Could you check a few things on this drawing? It's one solid part, dimensions in mm from its lowest x, y, z. A direction names the side the tool comes from. Give positions to 0.01 mm unless a question says otherwise; leave off trailing zeros. Loops run counter-clockwise (first coordinate to the right, second up) from the corner with the lowest first, then second, coordinate; pieces in that order, holes last. Notation, with made-up numbers: (29.25, 42) - (36.25, 42) arc R15 ccw to (36.25, 65) - close; hole circle Ø5 at (-22, 64.25). An arc over 180 degrees is marked (long way). Write item = value, one per line.
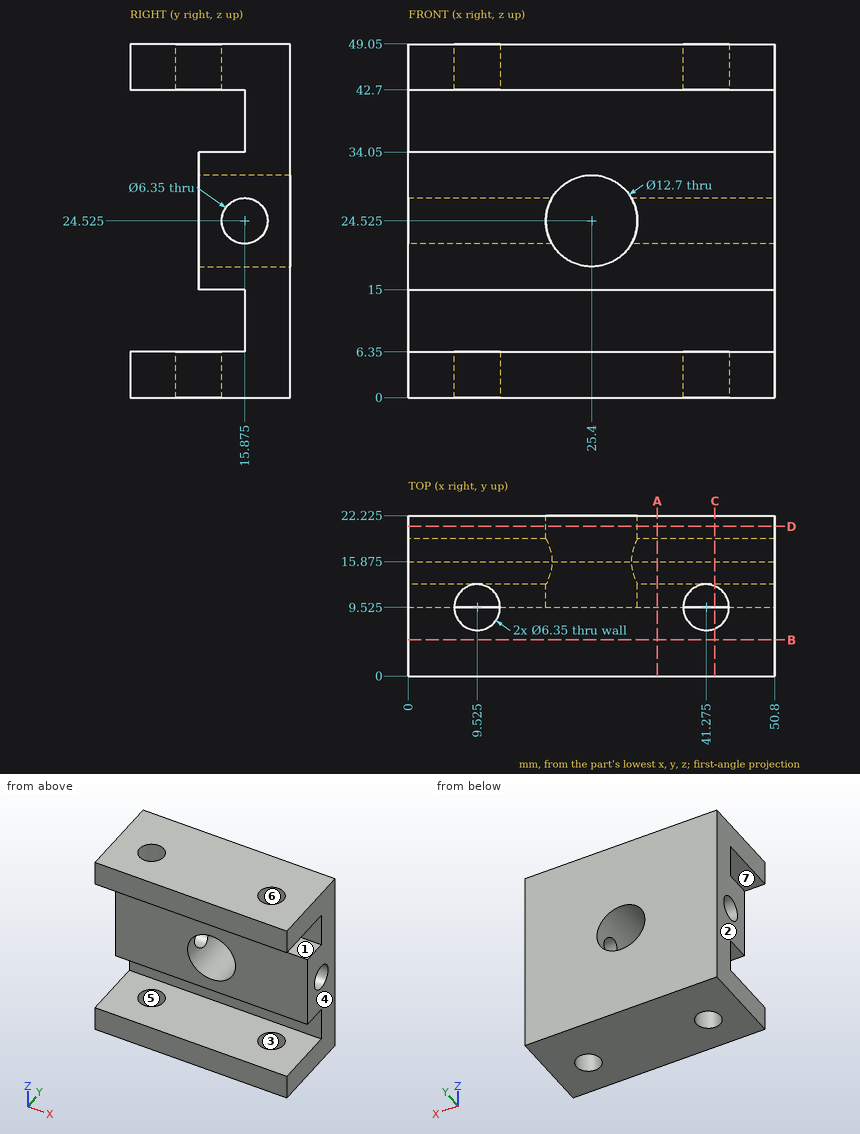
Q1. We'd pull the mould along X, two halves only. Please class the marked faces 1, 2, 3 and 4: released by +X, released by -X, zero draft, split by the parting line, or undercut.
Output:
face_1 = zero draft
face_2 = released by -X
face_3 = undercut
face_4 = released by +X
Q2. Imagine slicing it at B-B, the plane y = 5. Write out the boundary of the cut face in (x, z), then the cut area to 3 significant figures.
Output:
outline = (0, 0) - (50.8, 0) - (50.8, 6.35) - (0, 6.35) - close; (0, 42.7) - (50.8, 42.7) - (50.8, 49.05) - (0, 49.05) - close
area = 645 mm2
Q3. Which directions (+Z, -Z, +X, -X, +Y, -Y) give clear straight access to the entire face, cutting with the end or side of a thin tool? Please do the marked faces 5, 6 and 7.
Output:
face_5 = -Z
face_6 = +Z
face_7 = +X, -X, -Y
Q4. For pin 1 (4 mm diameter, centred on x = 41.275, y = 9.525, fed in from -Z); pin 2 (15 mm diameter, centred on x = 24.5, z = 27.5, fed in from -Y) (3 decimals); pin 3 (4.5 mm diameter, centred on x = 24.5, z = 38, fed in from -Y) (3 decimals), each with a flat end and sliding along its axis, tell me the tip position at first contact or that it passes through.
Output:
pin_1 = 15
pin_2 = 9.525
pin_3 = 15.875
Q5. Imagine slicing it at D-D, the plane y = 20.75. Write out the boundary of the cut face in (x, z) (3 decimals), then the cut area to 3 significant figures.
Output:
outline = (0, 0) - (50.8, 0) - (50.8, 49.05) - (0, 49.05) - close; hole circle Ø12.7 at (25.4, 24.525)
area = 2,370 mm2
Q6. I need wall thicknesses on L1, parallel to Z at x = 31.5, y = 5.75; L2, parallel to Z at x = 23.5, y = 10.75; L3, parallel to Z at x = 29.5, y = 12.25. Which ranges of each line are inside material? Lowest first, please.
Output:
L1 = 0 to 6.35, 42.7 to 49.05
L2 = 0 to 6.35, 15 to 18.47, 30.58 to 34.05, 42.7 to 49.05
L3 = 0 to 6.35, 15 to 19.68, 29.37 to 34.05, 42.7 to 49.05
Q7. Imagine slicing it at A-A, the plane x = 34.5. Write out the boundary of the cut face in (y, z) (3 decimals).
Output:
outline = (0, 0) - (22.225, 0) - (22.225, 49.05) - (0, 49.05) - (0, 42.7) - (15.875, 42.7) - (15.875, 34.05) - (9.525, 34.05) - (9.525, 15) - (15.875, 15) - (15.875, 6.35) - (0, 6.35) - close; hole circle Ø6.35 at (15.875, 24.525)
Q8. Imagine slicing it at C-C, the plane x = 42.5. Write out the boundary of the cut face in (y, z) (3 decimals).
Output:
outline = (0, 0) - (6.596, 0) - (6.596, 6.35) - (0, 6.35) - close; (0, 42.7) - (6.596, 42.7) - (6.596, 49.05) - (0, 49.05) - close; (9.525, 15) - (15.875, 15) - (15.875, 6.35) - (12.454, 6.35) - (12.454, 0) - (22.225, 0) - (22.225, 49.05) - (12.454, 49.05) - (12.454, 42.7) - (15.875, 42.7) - (15.875, 34.05) - (9.525, 34.05) - close; hole circle Ø6.35 at (15.875, 24.525)
